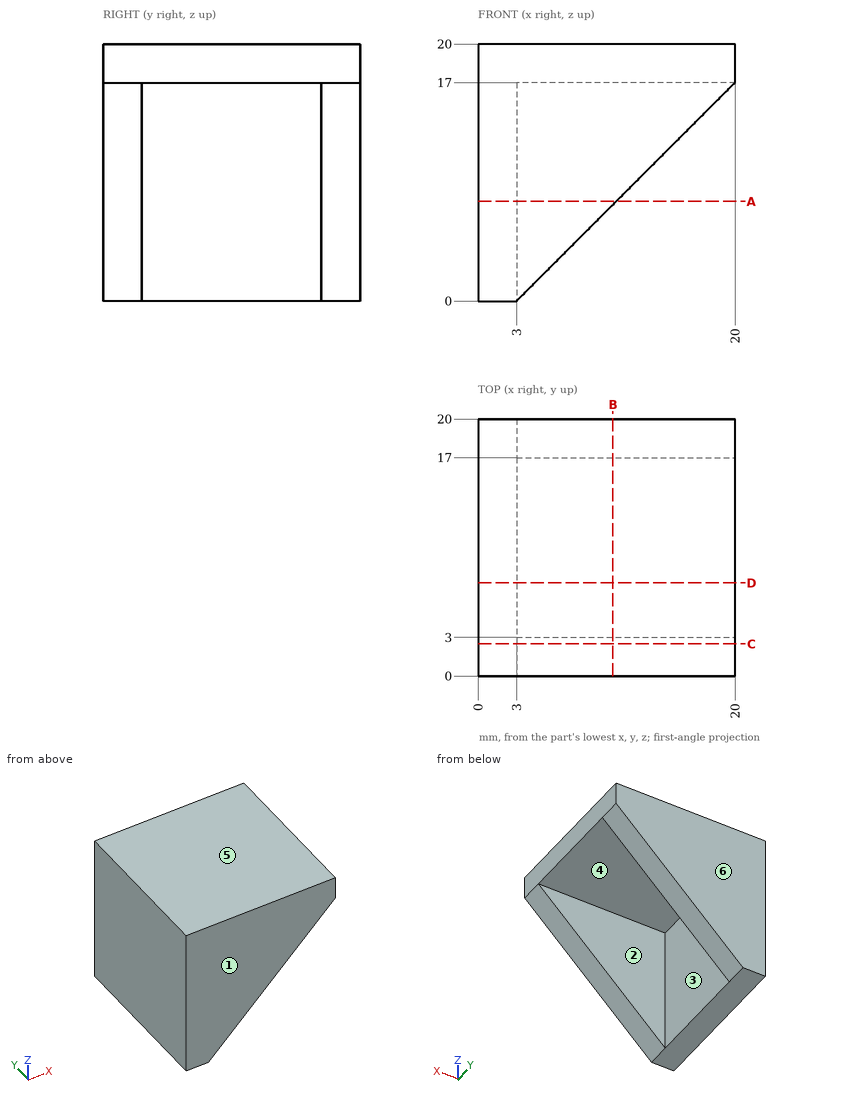
Source: three-view drawing plus pictorial views. Frame: mm from the lowest corner of the part. A direction names the side the tool comes from. Round coordinates to 2 decimals unless told otherwise and drop trailing zeros. Loops run counter-clockwise (first coordinate to the right, second up) from the corner with the lowest first, then second, coordinate; pieces in that order, holes last.
Q1. Section C-C on y = 2.5. Return loops of the section in (x, z), plus the area to 4 significant figures.
Q2. Material intervals for L1, parallel to Y at x = 10.25, z = 14.5; L2, parallel to X at y = 5.75, z = 5.75; L3, parallel to Z at x = 7, y = 12.75, sorted ascending.
Q3. Pin query (flat end, axial travel): P1, Ø4, axis at x = 8, y = 7.5, coming from the -Z side; P2, Ø12, axis at y = 4.5, z = 3, coming from the +X side; P3, Ø4, axis at y = 12, z = 6.5, coming from the +X side. Return the tip coordinate at first contact, or that it passes through.
Q4. Section A-A on z = 7.75. Return loops of the section in (x, y).
Q5. Section B-B on x = 10.5. Return loops of the section in (y, z).
Q6. Section D-D on y = 7.25. Return loops of the section in (x, z), plus the area to 3 significant figures.
Q7. Pull-direction query (Y, two-part tool) for the marked faces 3, 4, 5 and 6; classes: released by +Y, released by -Y, zero draft, split by the parting line, or undercut.
Q8. Access query for the marked faces 1 and 2. Directions: +Z, -Z, +X, -X, +Y, -Y. A direction counts if a zero-diameter tool reaches every point of the face in a straight line with its end or side. Return the directions, or none.
Evaluation:
1. outline: (0, 0) - (3, 0) - (20, 17) - (20, 20) - (0, 20) - close
1. area: 255.5 mm2
2. L1: y = 0 to 3, 17 to 20
2. L2: x = 0 to 3
2. L3: z = 17 to 20
3. P1: stops at z = 17
3. P2: stops at x = 11.81
3. P3: stops at x = 3
4. outline: (0, 0) - (10.75, 0) - (10.75, 3) - (3, 3) - (3, 17) - (10.75, 17) - (10.75, 20) - (0, 20) - close
5. outline: (0, 7.5) - (3, 7.5) - (3, 17) - (17, 17) - (17, 7.5) - (20, 7.5) - (20, 20) - (0, 20) - close
6. outline: (0, 0) - (3, 0) - (3, 17) - (20, 17) - (20, 20) - (0, 20) - close
6. area: 111 mm2
7. face 3: undercut
7. face 4: undercut
7. face 5: zero draft
7. face 6: released by +Y
8. face 1: +Z, -Z, +X, -X, -Y
8. face 2: -Z, +X
